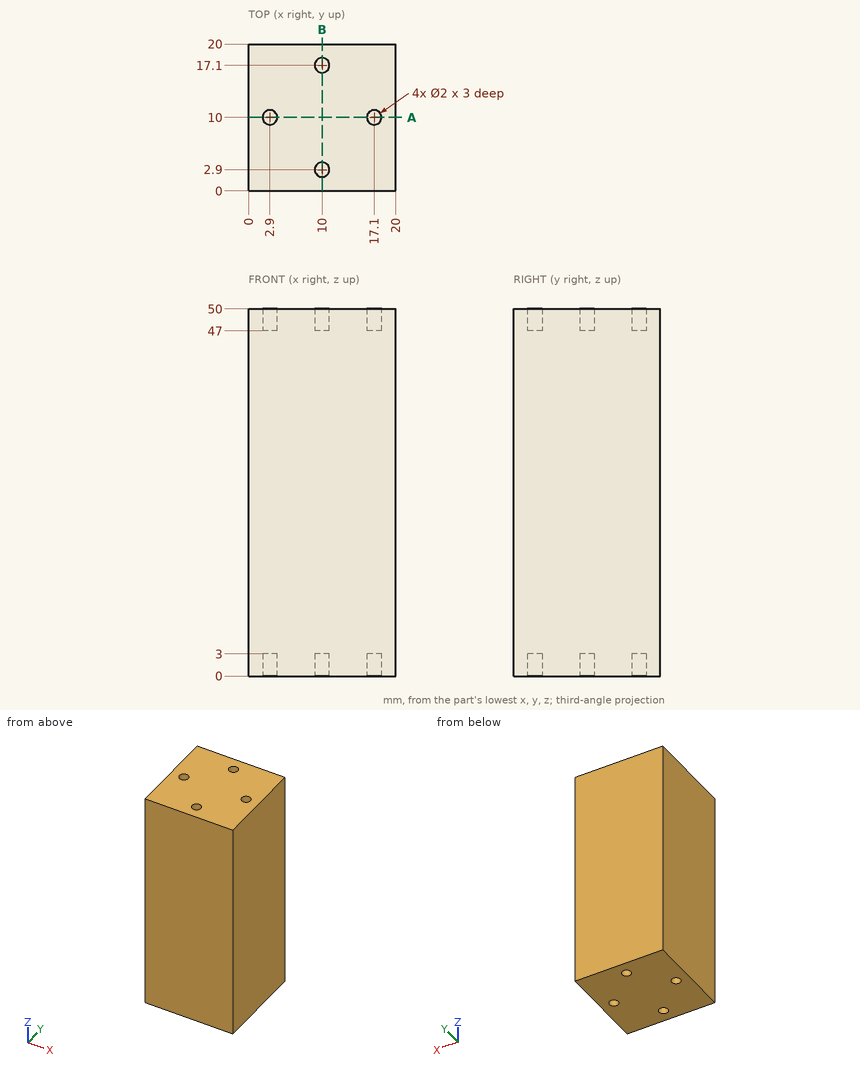
Verification items for this drawing (mm, ordinates from the low corner). Coordinates: 2 decimals unless noted, no trailing zeros. Loops run counter-clockwise (first coordinate to the right, second up) from the corner with the lowest first, then second, coordinate; pieces in that order, holes last. Notation, with made-up numbers: (-25, 81.5) - (28, 81.5) arc R21 cw to (28, 85.5) - close; hole circle Ø7 at (33.25, 79). An arc over 180 degrees is marked (long way). One line per item, written item: value. Start each with the question number.
(1) Cross-section at A-A on y = 10. Enter the section's corners in (x, z).
(2) Material ranges on line 1 (Y direction, x = 10, z = 48.65); line 2 (Y direction, x = 17.1, z = 47.8), recorded low to high. Write a range as [from, to].
(3) Depth check by flat-ended pin: P1, Ø1.8, axis at x = 17.1, y = 10, coming from the -Z side; P2, Ø1.2, axis at x = 10, y = 17.1, coming from the +Z side. Enter the tip coordinate at first touch or a pass-through.
Results below:
1. outline: (0, 0) - (1.9, 0) - (1.9, 3) - (3.9, 3) - (3.9, 0) - (16.1, 0) - (16.1, 3) - (18.1, 3) - (18.1, 0) - (20, 0) - (20, 50) - (18.1, 50) - (18.1, 47) - (16.1, 47) - (16.1, 50) - (3.9, 50) - (3.9, 47) - (1.9, 47) - (1.9, 50) - (0, 50) - close
2. line 1: y = [0, 1.9], [3.9, 16.1], [18.1, 20]
2. line 2: y = [0, 9], [11, 20]
3. P1: stops at z = 3
3. P2: stops at z = 47
